Verification items for the finished model (mm, model axes). Face numbers are marked on the shaded views. A direction names the side the tool comes from. Round coordinates to 2 decimals unless told otherwise and drop trailing zeros. Loops run counter-clockwise (first coordinate to the right, second up) from the corner with the lowest first, then second, coordinate; pieces in that order, holes last. Notation, with made-up numbers: M -6.5,-19.75 L 45.5,-19.75 A10 cw 45.5,-5.75 Z; hole C 89.5,72 d11. An arc over 180 degrees is marked long. Answer as CSV lines item,"result".
```python
from build123d import *

# Parameters (mm, degrees)
BOSS_EXTRUDE1_DEPTH = 60
SKETCH2_R           = 1.6
BOSS_EXTRUDE2_DEPTH = 4
CHAMFER1_SIZE       = 3
SKETCH3_R           = 1.6
CUT_EXTRUDE1_DEPTH  = 8
SKETCH4_R           = 1.6
CUT_EXTRUDE2_DEPTH  = 8
CHAMFER2_SIZE       = 10
CUT_EXTRUDE3_DEPTH  = 40


with BuildPart() as part:
    # Sketch1 → Boss-Extrude1 (new body)
    with BuildSketch(Plane.XY):
        Polygon((225, -175), (225, -135), (220, -135), (220, -172.928932188), (193.180194847, -199.748737342), (196.715728753, -203.284271247), align=None)
    extrude(amount=BOSS_EXTRUDE1_DEPTH)

    # Sketch2 → Boss-Extrude2 (add)
    with BuildSketch(Plane(origin=(0, 0, 0), x_dir=(-1, 0, 0), z_dir=(0, 0, -1))):
        Polygon((-225, -135), (-193.759605749, -135), (-174.625434131, -181.193976626), (-196.715728753, -203.284271247), (-225, -175), align=None)
        with Locations((-207.289508253, -167.664074122)):
            Circle(SKETCH2_R, mode=Mode.SUBTRACT)
        with Locations((-184.062077547, -179.316911543)):
            Circle(SKETCH2_R, mode=Mode.SUBTRACT)
        with Locations((-199.105034852, -143)):
            Circle(SKETCH2_R, mode=Mode.SUBTRACT)
    extrude(amount=-BOSS_EXTRUDE2_DEPTH)

    # Chamfer1
    chamfer1_edges = [part.edges().sort_by_distance(p)[0] for p in [
        (220, -153.964466094, 4),
        (206.590097423, -186.338834765, 4),
    ]]
    chamfer(chamfer1_edges, length=CHAMFER1_SIZE)

    # Sketch3 → Cut-Extrude1 (cut)
    with BuildSketch(Plane(origin=(225, 0, 0), x_dir=(0, 0, -1), z_dir=(1, 0, 0))):
        with Locations((-45, -150)):
            Circle(SKETCH3_R)
        with Locations((-15, -150)):
            Circle(SKETCH3_R)
    extrude(amount=-CUT_EXTRUDE1_DEPTH, mode=Mode.SUBTRACT)

    # Sketch4 → Cut-Extrude2 (cut)
    with BuildSketch(Plane(origin=(200, -200, 0), x_dir=(0, 0, -1), z_dir=(0.707106781, -0.707106781, 0))):
        with Locations((-45, 10.355339059)):
            Circle(SKETCH4_R)
        with Locations((-15, 10.355339059)):
            Circle(SKETCH4_R)
    extrude(amount=-CUT_EXTRUDE2_DEPTH, mode=Mode.SUBTRACT)

    # Chamfer2
    chamfer2_edges = [part.edges().sort_by_distance(p)[0] for p in [
        (222.5, -135, 60),
        (194.9479618, -201.516504294, 60),
    ]]
    chamfer(chamfer2_edges, length=CHAMFER2_SIZE)

    # Sketch5 → Cut-Extrude3 (cut)
    with BuildSketch(Plane(origin=(239.779220614, -99.319805153, 0), x_dir=(0, 0, -1), z_dir=(0.923879533, -0.382683432, 0))):
        Polygon((-37, -58.619964607), (-45, -66.619964607), (-45, -84.530327208), (-37, -92.530327208), (-4, -92.530327208), (-4, -58.619964607), align=None)
    extrude(amount=CUT_EXTRUDE3_DEPTH, mode=Mode.SUBTRACT)


solid = part.part
```
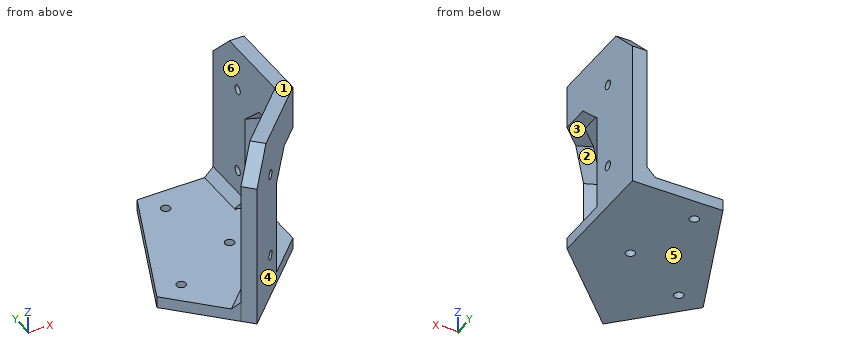
1) Set-up check for the marked faces 5 and 6: record each of +Z, -Z, +X, -X, +Y, -Y from which the full face is reachable in a straight line by a thin tool's end or side.
Here are the results:
face 5,"-Z, +X, -X, +Y, -Y"
face 6,"+Z, -X, +Y"
2) Draft check along Z on the marked faces 1, 2, 3 and 4. Enter one of: +Z half, -Z half, draft (parallel to the pull), parting line (faces both ways), or undercut.
Here are the results:
face 1,"+Z half"
face 2,"undercut"
face 3,"undercut"
face 4,"draft"
3) Section check D-D (x = 210). Record the cut outline in (y, z), plus the area to 3 significant figures.
Here are the results:
outline,"M -190,0 L -135,0 L -135,4 L -187.14,4 L -187.14,37 L -182.93,40.89 L -182.93,60 L -190,60 Z"
area,"469 mm^2"
4) Section check B-B (z = 15.5). Record the cut outline in (x, y), plus the area to 3 significant figures.
Here are the results:
outline,"M 193.18,-199.75 L 196.72,-203.28 L 206.25,-193.75 L 202.71,-190.22 Z; M 204.86,-188.07 L 208.4,-191.6 L 212.02,-187.98 L 207.02,-185.91 Z; M 220,-154.58 L 225,-156.65 L 225,-151.52 L 220,-151.52 Z; M 220,-148.48 L 225,-148.48 L 225,-135 L 220,-135 Z"
area,"176 mm^2"
5) Go/stop test with flat-tipped pins: pin 1 (8 mm diameter, centred on x = 196.5, y = -165.5, fed in from +Z); pin 2 (12 mm diameter, centred on x = 211.5, z = 13.5, fed in from -Y); pin 3 (10 mm diameter, centred on y = -152.5, z = 44.5, fed in from -X). Record where each tip stops, or that it passes through.
Here are the results:
pin 1,"stops at z = 4"
pin 2,"stops at y = -194.5"
pin 3,"stops at x = 220"
6) Section check C-C (y = -150). Record the cut outline in (x, z).
Here are the results:
outline,"M 187.55,0 L 225,0 L 225,13.4 L 220,13.4 L 220,7 L 217,4 L 187.55,4 Z; M 220,16.6 L 225,16.6 L 225,43.4 L 220,43.4 Z; M 220,46.6 L 225,46.6 L 225,60 L 220,60 Z"
7) Material ranges on probe 1 along Z at (x, y) = (222.6, -150); probe 2 along Z at (x, y) = (220.5, -178); probe 3 along Z at (x, y) = (213, -155), recorded low to high.
Here are the results:
probe 1,"z = 0 to 13.4, 16.6 to 43.4, 46.6 to 60"
probe 2,"z = 0 to 4, 45 to 60"
probe 3,"z = 0 to 4"
8) Section check A-A (y = -158). Record the cut outline in (x, z), plus the area to 3 significant figures.
Here are the results:
outline,"M 184.23,0 L 225,0 L 225,4 L 184.23,4 Z; M 220,40.16 L 225,38.25 L 225,60 L 220,60 Z"
area,"267 mm^2"
